```python
from build123d import *

# Parameters (mm, degrees)
F0_W          = 117.318443954
F0_H          = 54.2597807944
F1_DEPTH      = 3
F2_W          = 124.3039702
F2_H          = 60.2597807944
F2_W_2        = 117.318443954
F2_H_2        = 54.2597807944
F3_DEPTH      = 35
F4_R          = 5.9838878744
F5_DEPTH      = 35
F7_DEPTH      = 30.1308903972
F7_DEPTH_BACK = 30.1308903972


with BuildPart() as f1:
    # F0 (on Top) → F1 (new body)
    with BuildSketch(Plane.XY):
        Rectangle(F0_W, F0_H)
    extrude(amount=F1_DEPTH)

    # F2 (on Top) → F3 (join)
    with BuildSketch(Plane.XY):
        Rectangle(F2_W, F2_H)
        Rectangle(F2_W_2, F2_H_2, mode=Mode.SUBTRACT)
    extrude(amount=F3_DEPTH)

    # F4 (on Top) → F5 (join)
    with BuildSketch(Plane.XY):
        with Locations((-34.3156456947, 0)):
            Circle(F4_R)
        with Locations((34.3156456947, 0)):
            Circle(F4_R)
    extrude(amount=F5_DEPTH)

    # F6 (on Front) → F7 (cut, two sides)
    with BuildSketch(Plane.XZ) as f7_sk:
        with BuildLine():
            Line((18.4925086796, 35), (-18.4925086796, 35))
            Line((-18.4925086796, 35), (-18.4925086796, 22.2374610603))
            ThreePointArc((-18.4925086796, 22.2374610603), (0, 9.1160805646), (18.4925086796, 22.2374610603))
            Line((18.4925086796, 22.2374610603), (18.4925086796, 35))
        make_face()
    extrude(amount=-F7_DEPTH, mode=Mode.SUBTRACT)
    extrude(f7_sk.sketch, amount=F7_DEPTH_BACK, mode=Mode.SUBTRACT)


solid = f1.part
```
Verification items for the finished model (mm, model axes). A direction names the side the tool comes from. Coordinates: 2 decimals unless noted, no trailing zeros. Loops run counter-clockwise (first coordinate to the right, second up) from the corner with the lowest first, then second, coordinate; pieces in that order, holes last. Notation, with made-up numbers: (-39.5, -7) -> (-6.5, -7) arc R21 ccw to (-6.5, 2) -> close; hole circle Ø1 at (72, 77). An arc over 180 degrees is marked (long way). Put each result on its own line as item: value.
1. Section check B-B, the plane y = 0. Record the boundary of the cut face in (x, z).
Result set:
outline: (-62.15, 0) -> (62.15, 0) -> (62.15, 35) -> (58.66, 35) -> (58.66, 3) -> (40.3, 3) -> (40.3, 35) -> (28.33, 35) -> (28.33, 3) -> (-28.33, 3) -> (-28.33, 35) -> (-40.3, 35) -> (-40.3, 3) -> (-58.66, 3) -> (-58.66, 35) -> (-62.15, 35) -> close
2. Gauge pin test, flat end, axial feed: P1, Ø10, axis at x = -25, y = -19, coming from the +Z side. Record the tip position at first contact, or that the pin passes through.
Result set:
P1: stops at z = 3
3. Thickness scan on line 1 (X direction, y = 25.5, z = 6.5); line 2 (Y direction, x = 22, z = 31.5); line 3 (X direction, y = -2.5, z = 10). Record the ranges inside material, lowest first.
Result set:
line 1: x = -62.15 to -58.66, 58.66 to 62.15
line 2: y = -30.13 to -27.13, 27.13 to 30.13
line 3: x = -62.15 to -58.66, -39.75 to -28.88, 28.88 to 39.75, 58.66 to 62.15
4. Section check D-D, the plane z = 20. Record the boundary of the cut face in (x, y), then the cut area to 3 significant figures.
Result set:
outline: (-62.15, -30.13) -> (-17.55, -30.13) -> (-17.55, -27.13) -> (-58.66, -27.13) -> (-58.66, 27.13) -> (-17.55, 27.13) -> (-17.55, 30.13) -> (-62.15, 30.13) -> close; circle Ø11.97 at (-34.32, 0); (17.55, -30.13) -> (62.15, -30.13) -> (62.15, 30.13) -> (17.55, 30.13) -> (17.55, 27.13) -> (58.66, 27.13) -> (58.66, -27.13) -> (17.55, -27.13) -> close; circle Ø11.97 at (34.32, 0)
area: 1,140 mm^2
5. Tool access check on faces 1 (the face through (58.659, 0, 19)), 2 (the face through (-18.493, 29, 29)), 3 (the face through (60, 0, 35)). Record the directions out of +Z, -Z, +X, -X, +Y, -Y that give a thin tool (end or side, any length) a straight path to the whole face; none if there is none.
Result set:
face 1: +Z
face 2: +Z, +Y, -Y
face 3: +Z, +X, -X, +Y, -Y
6. Section check A-A, the plane z = 32.5. Record the boundary of the cut face in (x, y), then the cut area to 3 significant figures.
Result set:
outline: (-62.15, -30.13) -> (-18.49, -30.13) -> (-18.49, -27.13) -> (-58.66, -27.13) -> (-58.66, 27.13) -> (-18.49, 27.13) -> (-18.49, 30.13) -> (-62.15, 30.13) -> close; circle Ø11.97 at (-34.32, 0); (18.49, -30.13) -> (62.15, -30.13) -> (62.15, 30.13) -> (18.49, 30.13) -> (18.49, 27.13) -> (58.66, 27.13) -> (58.66, -27.13) -> (18.49, -27.13) -> close; circle Ø11.97 at (34.32, 0)
area: 1,130 mm^2
7. Section check C-C, the plane x = -31.5. Record the boundary of the cut face in (y, z).
Result set:
outline: (-30.13, 0) -> (30.13, 0) -> (30.13, 35) -> (27.13, 35) -> (27.13, 3) -> (5.28, 3) -> (5.28, 35) -> (-5.28, 35) -> (-5.28, 3) -> (-27.13, 3) -> (-27.13, 35) -> (-30.13, 35) -> close
8. Mould release check, pull along X, two halves, no side actions. Record for faces 4 (the face through (-60, 0, 35)), 5 (the face through (62.152, 0, 17)), 6 (the face through (-58.659, 0, 19)): pulls with the +X half, pulls with the -X half, needs draft (parallel to the pull), parting line crosses it, or undercut.
Result set:
face 4: needs draft
face 5: pulls with the +X half
face 6: undercut
